from build123d import *

# Parameters (mm, degrees)
F0_W     = 50
F0_H     = 50
F1_DEPTH = 100
F4_DEPTH = 50


with BuildPart() as f1:
    # F0 (on Top) → F1 (new body)
    with BuildSketch(Plane.XY):
        Rectangle(F0_W, F0_H)
    extrude(amount=F1_DEPTH)

    # F3 (on 3pt) → F4 (cut, symmetric)
    with BuildSketch(Plane(origin=(0, 0, 0), x_dir=(-0.7071067812, 0.7071067812, 0), z_dir=(0.7071067812, 0.7071067812, 0))):
        Polygon((10, 85), (5.9807621135, 100), (-5.9807621135, 100), (-10, 85), align=None)
        Polygon((45.3553390593, 85), (41.3361011729, 100), (29.3745769458, 100), (25.3553390593, 85), align=None)
        Polygon((-25.3553390593, 85), (-29.3745769458, 100), (-41.3361011729, 100), (-45.3553390593, 85), align=None)
    extrude(amount=F4_DEPTH, both=True, mode=Mode.SUBTRACT)


solid = f1.part
Build history of the part. All positions in model axes, mm. A direction names the side the tool comes from. Give positions to 0.01 mm unless a question says otherwise; leave off trailing zeros. Write each loop counter-clockwise with the first axis right and the second up, starting at its lowest first coordinate (ties: lowest second). Pieces come first, ordered by that corner, then holes. Notation, with made-up numbers: (27, -16) - (64, -16) arc R16 ccw to (64, 10) - close; hole circle Ø10 at (19, 45). An arc over 180 degrees is marked (long way). Use one line per item in the form item = value. Start each with the question number.
1. 3-axis set-ups, long thin cutter, end or side, ignore diameter. For faces 1 (the face through (0, 0, 85)), 2 (the face through (-19.47, 19.27, 92.6)), 3 (the face through (21, -21, 85)): which of +Z, -Z, +X, -X, +Y, -Y reach the whole face in a straight line?
2. Band-saw the part on A-A on y = 12. Write the cut outline in (x, z).
3. Probe line 1 (Z direction, x = -18, y = -10); line 2 (Y direction, x = -11, z = 87.5); line 3 (X direction, y = 0.5, z = 86.5). List the from-to ranges inside material, lowest first. Write a range as [from, to].
4. Band-saw the part on C-C on y = 6.5. Write the cut outline in (x, z), plus the area to 3 significant figures.
5. Two-plate mould, pull along Y, no slides. Class faces 4 (the face through (-5.96, 5.38, 92.4)), 5 (the face through (-21, 21, 85)), 6 (the face through (0, -25, 49)): released by +Y, released by -Y, zero draft, split by the parting line, or undercut.
6. Band-saw the part on B-B on x = -15. Write the cut outline in (y, z), plus the area to 3 significant figures.
Conclusion:
q1.face_1 = none
q1.face_2 = -X, +Y
q1.face_3 = +X, -Y
q2.outline = (-25, 0) - (25, 0) - (25, 85) - (-2.14, 85) - (3.54, 100) - (-25, 100) - (-25, 88.01) - (-23.86, 85) - (-25, 85) - close; (20.46, 100) - (25, 88.01) - (25, 100) - close
q3.line_1 = [0, 85]
q3.line_2 = [-25, -24.19], [2.19, 25]
q3.line_3 = [-25, -13.07], [14.07, 25]
q4.outline = (-25, 0) - (25, 0) - (25, 100) - (14.96, 100) - (20.64, 85) - (-7.64, 85) - (-1.96, 100) - (-25, 100) - close
q4.area = 4,660 mm²
q5.face_4 = undercut
q5.face_5 = zero draft
q5.face_6 = released by -Y
q6.outline = (-25, 0) - (25, 0) - (25, 85) - (20.86, 85) - (25, 95.93) - (25, 100) - (-6.54, 100) - (-0.86, 85) - (-25, 85) - close; (-25, 95.93) - (-23.46, 100) - (-25, 100) - close
q6.area = 4,660 mm²
